```python
from build123d import *

# Parameters (mm, degrees)
F0_R     = 4.0005
F1_DEPTH = 76.2
F2_R     = 4.0005
F3_ANGLE = 180


with BuildPart() as f1:
    # F0 (on Top) → F1 (new body)
    with BuildSketch(Plane.XY):
        Circle(F0_R)
    extrude(amount=F1_DEPTH)



with BuildPart() as f1b:
    # F0 (on Top) → F1, piece 2 (new body)
    with BuildSketch(Plane.XY):
        with Locations((-120.06, 0)):
            Circle(F0_R)
    extrude(amount=F1_DEPTH)


with BuildPart() as f1_1:
    add(f1.part)

    add(f1b.part)  # F3 merges F1b
    # F2 (on face) → F3 (revolve)
    with BuildSketch(Plane.XY.offset(76.2)):
        with Locations((-120.06, 0)):
            Circle(F2_R)
    revolve(axis=Axis((-60.03, -12.1569465846, 76.2), (0, 1, 0)), revolution_arc=F3_ANGLE)


solid = f1_1.part
```
Source: CAD feature listing. Evaluate the final solid. Frame: model axes, mm. Round coordinates to 2 decimals unless told otherwise and drop trailing zeros. Loops run counter-clockwise (first coordinate to the right, second up) from the corner with the lowest first, then second, coordinate; pieces in that order, holes last. Notation, with made-up numbers: M 55.5,2 L 80.5,2 A26 ccw 80.5,30 Z; hole C 38,27.5 d11. An arc over 180 degrees is marked long. Use a Markdown table: item, result. Add a question column.
1. Line query: line 1 (X direction, y = -1.25, z = 122.5); line 2 (X direction, y = -2.5, z = 35); line 3 (Z direction, x = -64, y = -3). Output: solid intervals per line, ascending.
2. Contact query for flat-ended pins moving along their axis: P1, Ø4, axis at x = -84.5, y = -2, coming from the +Z side; P2, Ø3, axis at y = 2, z = 93.5, coming from the +X side; P3, Ø8, axis at x = -88.5, z = 120.5, coming from the +Y side. Output: stop coordinate, or through.
3. Section query B-B on y = -2. Return the cut outline in (x, z), then the cut area to 3 significant figures.
4. Section query A-A on z = 13.5. Return the cut outline in (x, y), then the cut area to 3 significant figures.
5. Mould query, pull axis X, two halves, no side actions, for faces 1 (the cylindrical face through (-0.9, -3.9, 37.6)), 2 (the flat face through (0, 0, 0)), 3 (the cylindrical face through (-116.365, -1.532, 37.567)). Classes: pulls with the +X half, pulls with the -X half, needs draft (parallel to the pull), parting line crosses it, or undercut.
Reported:
| question | item | result |
|---|---|---|
| 1 | line 1 | x = -103.97 to -91.94, -28.12 to -16.09 |
| 1 | line 2 | x = -123.18 to -116.94, -3.12 to 3.12 |
| 1 | line 3 | z = 133.45 to 138.75 |
| 2 | P1 | stops at z = 135.92 |
| 2 | P2 | stops at x = 1.79 |
| 2 | P3 | stops at y = 2.16 |
| 3 | outline | M -123.52,0 L -116.6,0 L -116.6,76.2 A56.57 cw -3.46,76.2 L -3.46,0 L 3.46,0 L 3.46,76.2 A63.49 ccw -123.52,76.2 Z |
| 3 | area | 2,360 mm² |
| 4 | outline | C -120.06,0 d8; C 0,0 d8 |
| 4 | area | 101 mm² |
| 5 | face 1 | undercut |
| 5 | face 2 | needs draft |
| 5 | face 3 | undercut |
